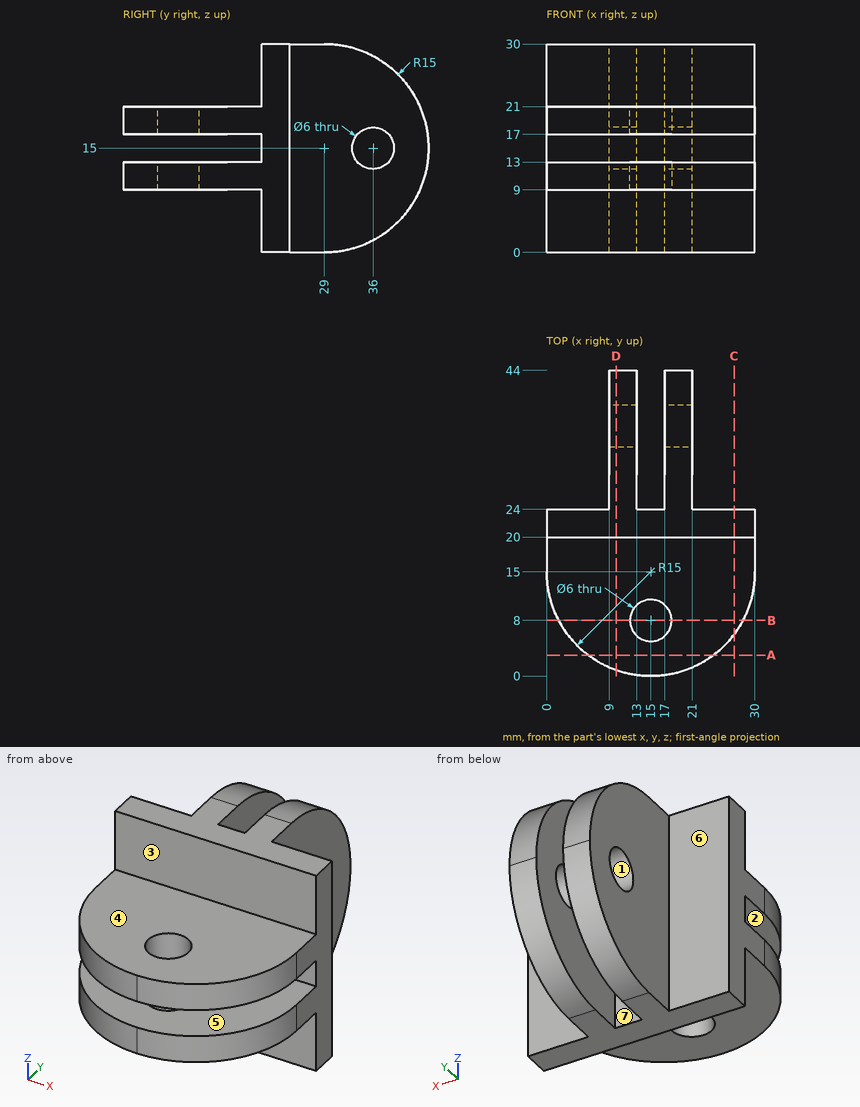
Input: dimensioned drawing with shaded views. Units: mm. Origin: part minimum x, y, z. A direction names the side the tool comes from. Coordinates: 2 decimals unless noted, no trailing zeros. Order: outer loops, then holes, each group sorted by start corner. A loop starts at its lowest first (then second) coordinate and runs counter-clockwise, first axis right, second up. Notation, with made-up numbers: (-7.75, -16) - (43.25, -16) arc R16 cw to (43.25, 13) - close; hole circle Ø9 at (-33.75, 64). An arc over 180 degrees is marked (long way). Return JSON: item names as keys, results as strings. Group by question number.
1. Pull-direction query (Y, two-part tool) for the marked faces 1, 2 and 3; classes: pulls with the +Y half, pulls with the -Y half, needs draft (parallel to the pull), parting line crosses it, or undercut.
2. Cut plane A-A (y = 3). Output: boundary loops of the cut face in (x, z).
3. Set-up query: the marked faces 4, 5, 6 and 7. Return all of +Z, -Z, +X, -X, +Y, -Y with unobstructed straight access to the full face (end or side cutting, diameter ignored); none if empty.
4. Cut plane C-C (x = 27). Output: boundary loops of the cut face in (y, z).
5. Material intervals for line 1 along X through (y, z) = (25, 25.5); line 2 along Y through (x, z) = (15.5, 25.5), sorted ascending. Write a range as [from, to].
6. Cut plane D-D (x = 10). Output: boundary loops of the cut face in (y, z), plus the area to 3 significant figures.
7. Cut plane B-B (y = 8). Output: boundary loops of the cut face in (x, z).
8. Pin query (flat end, axial travel): pin 1 (3 mm diameter, centred on x = 16, z = 15, fed in from -Y); pin 2 (4.5 mm diameter, centred on x = 24, z = 17.5, fed in from +Y); pin 3 (6 mm diameter, centred on y = 32.5, z = 9, fed in from -X). Return the tip coordinate at first contact, or that it passes through.
Resolved:
{
 "1": {"face 1": "undercut", "face 2": "needs draft", "face 3": "pulls with the -Y half"},
 "2": {"outline": "(6, 9) - (24, 9) - (24, 13) - (6, 13) - close; (6, 17) - (24, 17) - (24, 21) - (6, 21) - close"},
 "3": {"face 4": "+Z, +X, -X, -Y", "face 5": "+X, -X, -Y", "face 6": "+Z, -Z, -X, +Y", "face 7": "+Z, -Z, +Y"},
 "4": {"outline": "(6, 9) - (20, 9) - (20, 0) - (24, 0) - (24, 30) - (20, 30) - (20, 21) - (6, 21) - (6, 17) - (20, 17) - (20, 13) - (6, 13) - close"},
 "5": {"line 1": "x = [9, 13], [17, 21]", "line 2": "y = [20, 24]"},
 "6": {"outline": "(0.86, 9) - (20, 9) - (20, 0) - (29, 0) arc R15 ccw to (44, 15) arc R15 ccw to (29, 30) - (20, 30) - (20, 21) - (0.86, 21) - (0.86, 17) - (20, 17) - (20, 13) - (0.86, 13) - close; hole circle Ø6 at (36, 15)", "area": "748 mm²"},
 "7": {"outline": "(1.73, 9) - (12, 9) - (12, 13) - (1.73, 13) - close; (1.73, 17) - (12, 17) - (12, 21) - (1.73, 21) - close; (18, 9) - (28.27, 9) - (28.27, 13) - (18, 13) - close; (18, 17) - (28.27, 17) - (28.27, 21) - (18, 21) - close"},
 "8": {"pin 1": "stops at y = 20", "pin 2": "stops at y = 24", "pin 3": "stops at x = 9"}
}
